```python
from build123d import *

# Parameters (mm, degrees)
F1_DEPTH = 5
F2_R     = 4
F3_DEPTH = 30
F4_SIZE  = 1


with BuildPart() as f1:
    # F0 (on Top) → F1 (new body)
    with BuildSketch(Plane.XY):
        Polygon((3.464102, 6), (-3.464102, 6), (-6.928203, 0), (-3.464102, -6), (3.464102, -6), (6.928203, 0), align=None)
    extrude(amount=F1_DEPTH)

    # F2 (on face) → F3 (join)
    with BuildSketch(Plane(origin=(0, 0, 0), x_dir=(1, 0, 0), z_dir=(0, 0, -1))):
        Circle(F2_R)
    extrude(amount=F3_DEPTH)

    # F4
    f4_edges = [f1.edges().sort_by_distance(p)[0] for p in [
        (-4, 0, -30),
    ]]
    chamfer(f4_edges, length=F4_SIZE)


solid = f1.part
```
Design review of the part built by this model. Coordinates are the model's own, in mm. A direction names the side the tool comes from. Give positions to 0.01 mm unless a question says otherwise; leave off trailing zeros. Write each loop counter-clockwise with the first axis right and the second up, starting at its lowest first coordinate (ties: lowest second). Pieces come first, ordered by that corner, then holes.
(1) Clearance check with flat-ended pins moving along their axes: pin 1 Ø1.5 at (y, z) = (-1.5, -1.5) entering from +X; pin 2 Ø5 at (y, z) = (-2, -19.5) entering from +X. State where each tip first meets the part, or that it passes through.
Checked values:
pin 1: stops at x = 3.93
pin 2: stops at x = 4
(2) Add section B-B (z = -17). Give the boundary of the cut face in (x, y), and give its area (3 significant figures).
Checked values:
outline: circle Ø8 at (0, 0)
area: 50.3 mm2
(3) Wall thickness on line 1 along Z through (x, y) = (3.5, -5.25); line 2 along X through (y, z) = (0.25, -22); line 3 along X through (y, z) = (2, -19): over which ranges is each line inside the solid? List them lowest first.
Checked values:
line 1: z = 0 to 5
line 2: x = -3.99 to 3.99
line 3: x = -3.46 to 3.46
(4) Add section C-C (y = 5). Give the boundary of the cut face in (x, z), and give its area (3 significant figures).
Checked values:
outline: (-4.04, 0) - (4.04, 0) - (4.04, 5) - (-4.04, 5) - close
area: 40.4 mm2
(5) Add section D-D (z = 2). Give the boundary of the cut face in (x, y).
Checked values:
outline: (-6.93, 0) - (-3.46, -6) - (3.46, -6) - (6.93, 0) - (3.46, 6) - (-3.46, 6) - close
(6) Add section A-A (x = 0). Give the boundary of the cut face in (y, z).
Checked values:
outline: (-6, 0) - (-4, 0) - (-4, -29) - (-3, -30) - (3, -30) - (4, -29) - (4, 0) - (6, 0) - (6, 5) - (-6, 5) - close
(7) Tool access review of faces 1 (the face through (0, 0, 5)), 2 (the face through (-0.867, 3.905, -14.297)): name each direction out of +Z, -Z, +X, -X, +Y, -Y from which nothing blocks a thin tool from reaching the whole face with its end or side.
Checked values:
face 1: +Z, +X, -X, +Y, -Y
face 2: -Z
